```python
from build123d import *

# Parameters (mm, degrees)
F1_DEPTH = 25.4
F0_R     = 12.7
F2_DEPTH = 25.4


# Not quite as in the source:
# - the program builds the solid bodies; features that only make, move or delete a surface that nothing else refers to are left out


with BuildPart() as f1:
    # F0 (on Front) → F1 (new body)
    with BuildSketch(Plane.XZ):
        with BuildLine():
            Line((12.1809959468, 31.3732746576), (0, 33.655))
            ThreePointArc((0, 33.655), (-33.498646558, -3.2403246414), (6.4505416667, -33.0310389968))
            ThreePointArc((6.4505416667, -33.0310389968), (25.9783756689, -21.3958646146), (33.655, 0))
            ThreePointArc((33.655, 0), (27.7723823572, 19.0093083305), (12.1809959468, 31.3732746576))
        make_face()
        with BuildLine():
            ThreePointArc((-11.7732150983, 4.7625), (0, 12.7), (11.7732150983, 4.7625))
            Line((11.7732150983, 4.7625), (19.05, 4.7625))
            Line((19.05, 4.7625), (19.05, -4.7625))
            Line((19.05, -4.7625), (11.7732150983, -4.7625))
            ThreePointArc((11.7732150983, -4.7625), (0, -12.7), (-11.7732150983, -4.7625))
            Line((-11.7732150983, -4.7625), (-19.05, -4.7625))
            Line((-19.05, -4.7625), (-19.05, 4.7625))
            Line((-19.05, 4.7625), (-11.7732150983, 4.7625))
        make_face(mode=Mode.SUBTRACT)
    extrude(amount=F1_DEPTH)

    # F0 (on Front) → F2 (join)
    with BuildSketch(Plane.XZ):
        with BuildLine():
            Line((12.1809959468, 31.3732746576), (0, 33.655))
            ThreePointArc((0, 33.655), (-33.498646558, -3.2403246414), (6.4505416667, -33.0310389968))
            ThreePointArc((6.4505416667, -33.0310389968), (25.9783756689, -21.3958646146), (33.655, 0))
            ThreePointArc((33.655, 0), (27.7723823572, 19.0093083305), (12.1809959468, 31.3732746576))
        make_face()
        with BuildLine():
            ThreePointArc((-11.7732150983, 4.7625), (0, 12.7), (11.7732150983, 4.7625))
            Line((11.7732150983, 4.7625), (19.05, 4.7625))
            Line((19.05, 4.7625), (19.05, -4.7625))
            Line((19.05, -4.7625), (11.7732150983, -4.7625))
            ThreePointArc((11.7732150983, -4.7625), (0, -12.7), (-11.7732150983, -4.7625))
            Line((-11.7732150983, -4.7625), (-19.05, -4.7625))
            Line((-19.05, -4.7625), (-19.05, 4.7625))
            Line((-19.05, 4.7625), (-11.7732150983, 4.7625))
        make_face(mode=Mode.SUBTRACT)
        with BuildLine():
            ThreePointArc((12.1809959468, 31.3732746576), (6.1964290683, 33.0796507207), (0, 33.655))
            Line((0, 33.655), (12.1809959468, 31.3732746576))
        make_face()
        with BuildLine():
            ThreePointArc((33.655, 0), (25.9783756689, -21.3958646146), (6.4505416667, -33.0310389968))
            Line((6.4505416667, -33.0310389968), (79.85125, -18.6968145265))
            ThreePointArc((79.85125, -18.6968145265), (57.1501407243, -0.0732227913), (79.7074126802, 18.7243305966))
            Line((79.7074126802, 18.7243305966), (12.1809959468, 31.3732746576))
            ThreePointArc((12.1809959468, 31.3732746576), (27.7723823572, 19.0093083305), (33.655, 0))
        make_face()
        with BuildLine():
            ThreePointArc((79.7074126802, 18.7243305966), (57.1501407243, -0.0732227913), (79.85125, -18.6968145265))
            ThreePointArc((79.85125, -18.6968145265), (90.9047409447, -12.110866763), (95.25, 0))
            ThreePointArc((95.25, 0), (90.8580815859, 12.167298148), (79.7074126802, 18.7243305966))
        make_face()
        with Locations((76.2, 0)):
            Circle(F0_R, mode=Mode.SUBTRACT)
    extrude(amount=F2_DEPTH)


solid = f1.part
```
Geometry check sheet. Reference: the model listing, model coordinates, mm. A direction names the side the tool comes from. Give positions to 0.01 mm unless a question says otherwise; leave off trailing zeros. Order: outer loops, then holes, each group sorted by start corner. A loop starts at its lowest first (then second) coordinate and runs counter-clockwise, first axis right, second up. Notation, with made-up numbers: (1.5, 21.25) -> (10.5, 21.25) arc R10 cw to (10.5, 28.25) -> close; hole circle Ø6 at (89, 78.25). An arc over 180 degrees is marked (long way). Write each question's results on one line, items separated by ' | '. Start each with the question number.
(1) Scan lines: line 1 (X direction, y = -12, z = 8.5); line 2 (X direction, y = -20.75, z = 3.5); line 3 (Z direction, x = 76.2, y = -8.5). Record each from-to range of solid material in increasing order.
(2) Sectioned sample at A-A (y = -3.25). Give the number of separate pieces and of enclosed holes in the cut face, plus the area to 3 significant figures.
(3) Mould release check, pull along X, two halves, no side actions. Record for faces 1 (the face through (30, 0, 0)), 2 (the face through (42.637, -12.522, -25.964)), 3 (the face through (-15, -13, 4.762)): pulls with the +X half, pulls with the -X half, needs draft (parallel to the pull), parting line crosses it, or undercut.
(4) Access from +Z, -Z, +X, -X, +Y, -Y to the whole of each face (thin tool, end or side, straight path). Record for faces 4 (the face through (46.42, -12.52, 24.96)), 5 (the face through (-19.05, -13, 0)).
(5) Sectioned sample at B-B (x = 17). Enter the section's corners in (y, z), plus the area to 3 significant figures.
(6) Gauge pin test, flat ends, axial feed: P1, Ø8, axis at x = 65, y = -6.5, coming from the -Z side; P2, Ø2, axis at x = 74.5, y = -14, coming from the +Z side; P3, Ø4, axis at x = 4, y = -5, coming from the -Z side. Record the tip position at first contact, or that the pin passes through.
(7) Sectioned sample at C-C (z = -3). Enter the section's corners in (x, y).
(8) Sectioned sample at D-D (x = 76.2). Enter the section's corners in (y, z).
Answer below:
1) line 1: -32.56 to -9.44, 9.44 to 66.76, 85.64 to 93.25 | line 2: -33.47 to -19.05, 19.05 to 63.99, 88.41 to 94.93 | line 3: -19.41 to -12.7, 12.7 to 19.38
2) separate pieces: 1 | enclosed holes: 2 | area: 5,280 mm2
3) face 1: needs draft | face 2: pulls with the +X half | face 3: undercut
4) face 4: +Z, +X, +Y, -Y | face 5: +Y, -Y
5) outline: (-25.4, -30.97) -> (0, -30.97) -> (0, -4.76) -> (-25.4, -4.76) -> close; (-25.4, 4.76) -> (0, 4.76) -> (0, 30.47) -> (-25.4, 30.47) -> close | area: 1,320 mm2
6) P1: z = -22.38 | P2: z = 19.89 | P3: z = -33.6
7) outline: (-33.52, -25.4) -> (-19.05, -25.4) -> (-19.05, 0) -> (-33.52, 0) -> close; (19.05, -25.4) -> (63.86, -25.4) -> (63.86, 0) -> (19.05, 0) -> close; (88.54, -25.4) -> (95.01, -25.4) -> (95.01, 0) -> (88.54, 0) -> close
8) outline: (-25.4, -19.41) -> (0, -19.41) -> (0, -12.7) -> (-25.4, -12.7) -> close; (-25.4, 12.7) -> (0, 12.7) -> (0, 19.38) -> (-25.4, 19.38) -> close
